For this review, take the finished solid that the model builds, in its own axes (mm). Face numbers are marked on the shaded views. A direction names the side the tool comes from. Coordinates: 2 decimals unless noted, no trailing zeros. Write each loop counter-clockwise with the first axis right and the second up, starting at its lowest first coordinate (ties: lowest second). Pieces come first, ordered by that corner, then holes. Notation, with made-up numbers: (-18, 73.25) - (-14, 73.25) arc R16 ccw to (-14, 82.25) - close; hole circle Ø4 at (79.25, 39.5). An arc over 180 degrees is marked (long way). Write each question's results on one line, items separated by ' | '.
from build123d import *

# Parameters (mm, degrees)
F1_DEPTH = 15
F2_W     = 8
F2_H     = 50
F3_DEPTH = 15
F4_W     = 20
F4_H     = 4
F5_DEPTH = 30


with BuildPart() as f1:
    # F0 (on Top) → F1 (new body)
    with BuildSketch(Plane.XY):
        with BuildLine():
            ThreePointArc((-240, 20), (-260, 0), (-240, -20))
            Line((-240, -20), (240, -20))
            ThreePointArc((240, -20), (260, 0), (240, 20))
            add(Edge.make_bspline(
                [(-240, 20), (-201.0380044732, 35.6526101303), (-111.5188369016, 71.6160819761), (127.7105565079, 78.2594773928), (206.7294289612, 37.2618727193), (240, 20)],
                knots=[0, 0, 0, 0, 0.3085194424, 0.7088549571, 1, 1, 1, 1], degree=3))
        make_face()
    extrude(amount=F1_DEPTH)

    # F2 (on Right) → F3 (join, symmetric)
    with BuildSketch(Plane.YZ):
        with BuildLine():
            Line((63.6485348786, 15), (71.6485348786, 15))
            add(Edge.make_bspline(
                [(71.6485348786, 15), (81.1055550979, 21.2851513885), (99.9699154527, 46.3766770593), (84.9787602317, 86.8551220677), (71.6485385144, 95)],
                knots=[0, 0, 0, 0, 0.4642688731, 1, 1, 1, 1], degree=3))
            Line((71.6485385144, 95), (63.6485385144, 95))
            add(Edge.make_bspline(
                [(63.6485385144, 95), (75.6313007905, 86.8630942273), (92.9907729816, 45.3965691415), (73.9991203582, 22.623041553), (63.6485348786, 15)],
                knots=[0, 0, 0, 0, 0.53596906, 1, 1, 1, 1], degree=3))
        make_face()
        with Locations((67.6485385144, 120)):
            Rectangle(F2_W, F2_H)
    extrude(amount=F3_DEPTH, both=True)

    # F4 (on face) → F5 (cut)
    with BuildSketch(Plane.XY.offset(145)):
        with Locations((0, 67.6485385144)):
            Rectangle(F4_W, F4_H)
    extrude(amount=-F5_DEPTH, mode=Mode.SUBTRACT)


solid = f1.part
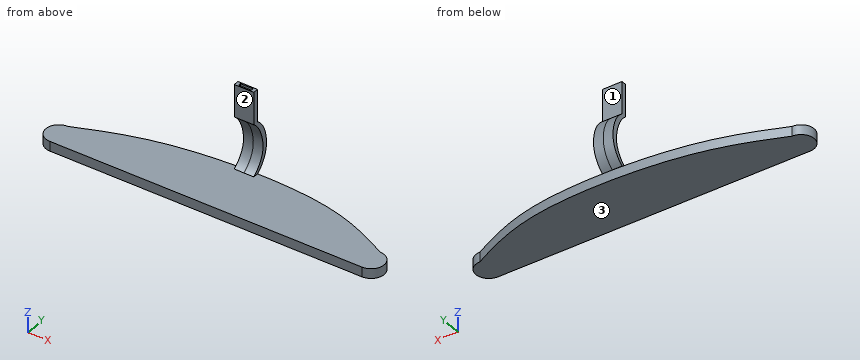
Q1. For pin 1 (4.5 mm diameter, centred on y = 67.5, z = 136.5, fed in from -X); pin 2 (10 mm diameter, centred on x = 5, z = 124, fed in from +Y); pin 3 (1.2 mm diameter, centred on y = 67.5, z = 133.5, fed in from +X), all flat-tipped, find the tip position at first contact; note any pin that passes through.
Results found:
pin 1: x = -15 | pin 2: y = 71.65 | pin 3: x = 15
Q2. Wall thickness on line 1 along Z through (x, y) = (-72.5, 21.5); line 2 along X through (y, z) = (84.5, 50); line 3 along Y through (x, z) = (-168.5, 8.5): over which ranges is each line inside the solid? List them lowest first. Write a range as from..to.
Results found:
line 1: 0..15 | line 2: -15..15 | line 3: -20..46.31
Q3. For the marked faces 1, 2 and 3, list the 3-axis set-ups (+Z, -Z, +X, -X, +Y, -Y) from which the entire face can be reached by the end or side of a thin tool; tool diameter is ignored.
Results found:
face 1: +Z, +X, -X, +Y | face 2: +Z, +X, -X, -Y | face 3: -Z, +X, -X, +Y, -Y
Q4. Take a section at A-A on z = 125.5. State the section outline as (x, y) points, plus the area to 3 significant figures.
Results found:
outline: (-15, 63.65) - (15, 63.65) - (15, 71.65) - (-15, 71.65) - close; hole (-10, 65.65) - (10, 65.65) - (10, 69.65) - (-10, 69.65) - close | area: 160 mm2
Q5. Take a section at B-B on y = 0. State the section outline as (x, z) points.
Results found:
outline: (-260, 0) - (260, 0) - (260, 15) - (-260, 15) - close
